Geometry: see drawing. Coordinates: mm, zero at the bounding-box minimum. A direction names the side the tool comes from. Give positions to 0.01 mm unless a question says otherwise; leave off trailing zeros. Order: outer loops, then holes, each group sorted by start corner. A loop starts at its lowest first (then second) coordinate and runs counter-clockwise, first axis right, second up. Notation, with made-up numbers: (87, 79.5) - (145, 79.5) arc R15 cw to (145, 98.5) - close; hole circle Ø6 at (62.5, 14.25). An arc over 180 degrees is marked (long way). Write each question's results on one line, items separated by ' | '. Start each with the question number.
Item 1: Contact query for flat-ended pins moving along their axis: pin 1 Ø4 at (y, z) = (6, 9) entering from +X; pin 2 Ø7 at (x, z) = (23.5, 1.5) entering from -Y; pin 3 Ø4 at (y, z) = (18, 4) entering from -X; pin 4 Ø1.4 at (x, z) = (1.5, 9) entering from +Y. Output: stop coordinate, or through.
Item 2: Line query: line 1 along X through (y, z) = (2.9, 6.25); line 2 along Y through (x, z) = (10, 2.5); line 3 along X through (y, z) = (20.5, 10.75). Output: solid intervals per line, ascending.
Item 3: Section A-A on x = 14.2. Output: boundary loops of the cut face in (y, z), and give its area (4 significant figures).
Item 4: Section B-B on y = 4.25. Output: boundary loops of the cut face in (x, z), and give its area (3 significant figures).
Item 5: Section D-D on y = 24. Output: boundary loops of the cut face in (x, z).
Item 6: Section C-C on z = 10.25. Output: boundary loops of the cut face in (x, y), and give its area (3 significant figures).
Item 7: Set-up query: the marked faces 4, 5 and 6. Return all of +Z, -Z, +X, -X, +Y, -Y with unobstructed straight access to the full face (end or side cutting, diameter ignored); none if empty.
Item 8: Mould query, pull axis X, two halves, no side actions, for the marked faces 1, 2 and 3. Classes: released by +X, released by -X, zero draft, split by the parting line, or undercut.
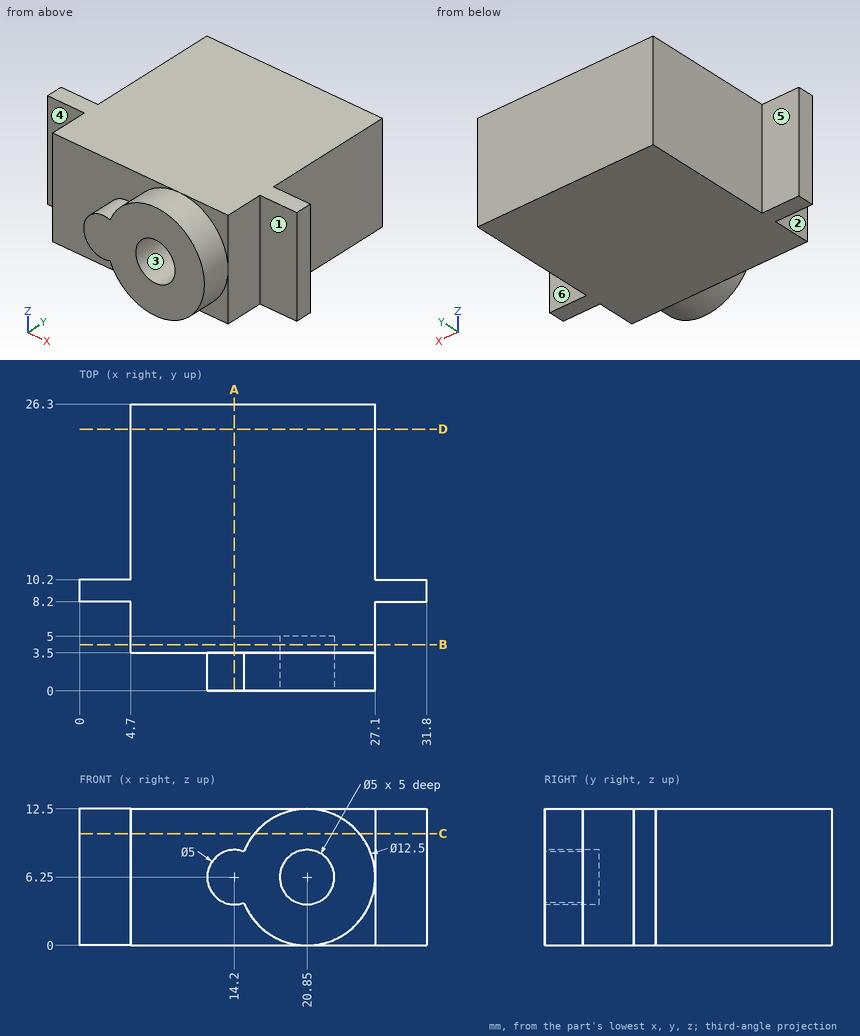
Evaluation:
1) pin 1: stops at x = 27.1 | pin 2: stops at y = 0 | pin 3: stops at x = 4.7 | pin 4: stops at y = 10.2
2) line 1: x = 11.7 to 18.35, 23.35 to 27.1 | line 2: y = 3.5 to 26.3 | line 3: x = 4.7 to 27.1
3) outline: (0, 3.75) - (3.5, 3.75) - (3.5, 0) - (26.3, 0) - (26.3, 12.5) - (3.5, 12.5) - (3.5, 8.75) - (0, 8.75) - close | area: 302.5 mm^2
4) outline: (4.7, 0) - (27.1, 0) - (27.1, 12.5) - (4.7, 12.5) - close; hole circle Ø5 at (20.85, 6.25) | area: 260 mm^2
5) outline: (4.7, 0) - (27.1, 0) - (27.1, 12.5) - (4.7, 12.5) - close
6) outline: (0, 8.2) - (4.7, 8.2) - (4.7, 3.5) - (16.05, 3.5) - (16.05, 0) - (25.65, 0) - (25.65, 3.5) - (27.1, 3.5) - (27.1, 8.2) - (31.8, 8.2) - (31.8, 10.2) - (27.1, 10.2) - (27.1, 26.3) - (4.7, 26.3) - (4.7, 10.2) - (0, 10.2) - close | area: 563 mm^2
7) face 4: +Z, -Z, -X, -Y | face 5: +Z, -Z, -X, +Y | face 6: +Z, -Z, +X, +Y
8) face 1: zero draft | face 2: released by -X | face 3: undercut
